The figure shows three views and two pictorial views of one solid part (mm, origin at its lowest corner). Answer the questions. A direction names the side the tool comes from. Coordinates: 2 decimals unless noted, no trailing zeros. Write each loop counter-clockwise with the first axis right and the second up, starting at its lowest first coordinate (ties: lowest second). Pieces come first, ordered by that corner, then holes. Notation, with made-up numbers: M 41.5,32.25 L 100.5,32.25 A12 cw 100.5,39.25 Z; hole C -20,52.5 d10. An arc over 180 degrees is marked long. Answer as CSV lines item,"result".
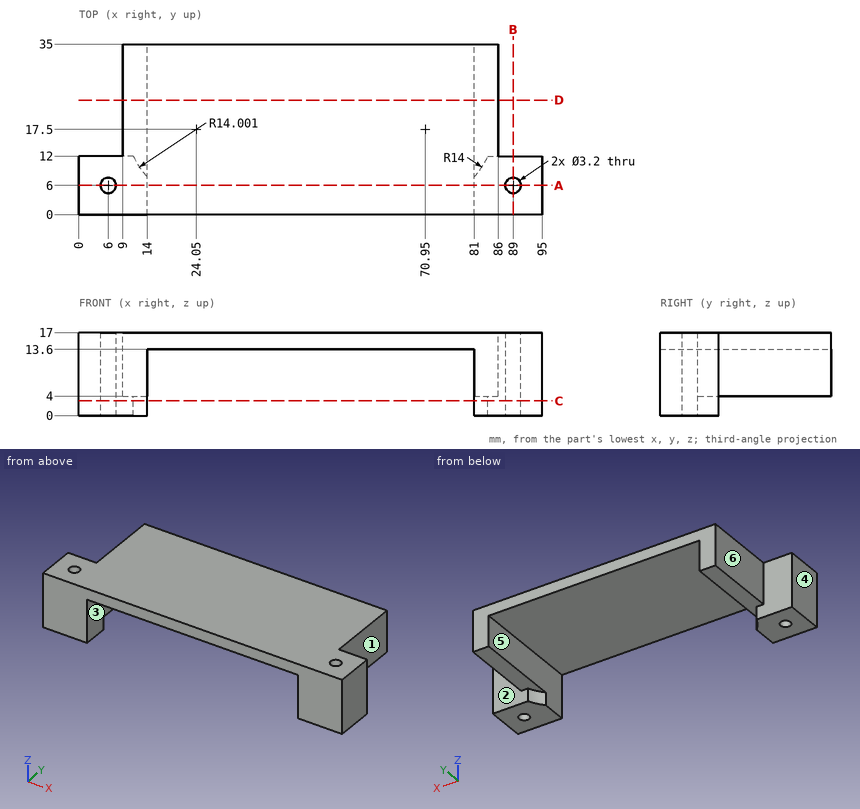
Q1. Find section A-A (y = 6). Give the vertices of the cut face in (x, z).
Output:
outline,"M 0,0 L 4.4,0 L 4.4,17 L 0,17 Z; M 7.6,0 L 14,0 L 14,13.6 L 81,13.6 L 81,0 L 87.4,0 L 87.4,17 L 7.6,17 Z; M 90.6,0 L 95,0 L 95,17 L 90.6,17 Z"
Q2. Find section D-D (y = 23.5). Give the vertices of the cut face in (x, z).
Output:
outline,"M 9,4 L 14,4 L 14,13.6 L 81,13.6 L 81,4 L 86,4 L 86,17 L 9,17 Z"
Q3. Flat-ended cylindrical pins translate along their axes: pin 1 Ø2.5 at (x, y) = (11, 17.5) entering from -Z; pin 2 Ø17.5 at (x, y) = (36.5, 24) entering from -Z; pin 3 Ø4 at (y, z) = (20, 9) entering from -X. Find the tip coordinate at first contact, or state that the pin passes through.
Output:
pin 1,"z = 4"
pin 2,"z = 13.6"
pin 3,"x = 9"
Q4. Straight lines are drawn through the part: line 1 (X direction, y = 6, z = 5.5); line 2 (X direction, y = 29, z = 5); line 3 (Y direction, x = 6, z = 5.5). For each, find the intervals that lie inside material, in ascending order.
Output:
line 1,"0 to 4.4, 7.6 to 14, 81 to 87.4, 90.6 to 95"
line 2,"9 to 14, 81 to 86"
line 3,"0 to 4.4, 7.6 to 12"
Q5. Find section C-C (z = 3). Count the separate pieces of the cut face and the enclosed holes in it, and give its area (3 significant figures).
Output:
separate pieces,"2"
enclosed holes,"2"
area,"306 mm2"
Q6. For the marked faces 4, 5 and 6, determine the directions among +Z, -Z, +X, -X, +Y, -Y from which every point of the face is accessible in a straight line to the end or side of a thin tool.
Output:
face 4,"+Z, -Z, -X, +Y, -Y"
face 5,"-Z, +Y, -Y"
face 6,"+Z, -Z, -X, +Y"
Q7. Find section B-B (x = 89). Give the vertices of the cut face in (y, z), and give its area (3 significant figures).
Output:
outline,"M 0,0 L 4.4,0 L 4.4,17 L 0,17 Z; M 7.6,0 L 12,0 L 12,17 L 7.6,17 Z"
area,"150 mm2"
Q8. The mould has two halves that part along X. Classify the marked faces 1, 2 and 3: pulls with the +X half, pulls with the -X half, needs draft (parallel to the pull), parting line crosses it, or undercut.
Output:
face 1,"pulls with the +X half"
face 2,"needs draft"
face 3,"undercut"
